from build123d import *

# Parameters (mm, degrees)
CHAMFER1_SIZE    = 0.79375
CHAMFER1_SIZE2   = 3.175
EXTRUSION1_DEPTH = 3.175
ESQUISSE3_R      = 9.165435523
EXTRUSION2_DEPTH = 1.5875
ESQUISSE4_R      = 6.5786
THREAD1_DEPTH    = 4.7625
CHAMFER2_SIZE    = 0.79375
HOLE1_D          = 10.16


with BuildPart() as part:
    # Esquisse1 → Revolution1 (revolve)
    with BuildSketch(Plane.XY, mode=Mode.PRIVATE) as revolution1_sk:
        Polygon((0, 5.08), (19.05, 5.08), (19.05, 6.477), (15.24, 6.477), (15.24, 5.842), (12.7, 6.477), (12.7, 5.842), (10.16, 6.477), (10.16, 5.842), (7.62, 6.477), (7.62, 5.842), (5.08, 6.477), (4.7625, 6.477), (4.7625, 5.842), (0, 5.842), align=None)
    revolve(revolution1_sk.sketch.rotate(Axis((0, 0, 0), (1, 0, 0)), 90), axis=Axis((0, 0, 0), (1, 0, 0)))

    # Chamfer1
    chamfer1_edges = [part.edges().sort_by_distance(p)[0] for p in [
        (19.05, 0, -6.477),
    ]]
    chamfer1_side = [part.faces().sort_by_distance(p)[0] for p in [
        (19.05, 0, -5.263197225),
    ]]
    chamfer(chamfer1_edges, length=CHAMFER1_SIZE, length2=CHAMFER1_SIZE2, reference=chamfer1_side[0])

    # Esquisse2 → Extrusion1 (add)
    with BuildSketch(Plane.ZY):
        Polygon((0.375877143, -9.157724865), (-7.742883803, -4.904381587), (-8.118760946, 4.253343278), (-0.375877143, 9.157724865), (7.742883803, 4.904381587), (8.118760946, -4.253343278), align=None)
    extrude(amount=EXTRUSION1_DEPTH)

    # Esquisse3 → Extrusion2 (add)
    with BuildSketch(Plane.ZY.offset(3.175)):
        with Locations(Location((0, 0, 0), (0, 0, 152.350375514))):
            Circle(ESQUISSE3_R)
    extrude(amount=EXTRUSION2_DEPTH)

    # Esquisse4 → Thread1 (add)
    with BuildSketch(Plane.ZY.offset(4.7625)):
        with Locations(Location((0, 0, 0), (0, 0, 180))):
            Circle(ESQUISSE4_R)
    extrude(amount=THREAD1_DEPTH)

    # Chamfer2
    chamfer2_edges = [part.edges().sort_by_distance(p)[0] for p in [
        (-9.525, 0, 6.5786),
    ]]
    chamfer(chamfer2_edges, length=CHAMFER2_SIZE)

    # Hole1 (through all)
    with Locations(Plane.ZY.offset(9.525)):
        with Locations((0, 0)):
            Hole(HOLE1_D / 2)


solid = part.part
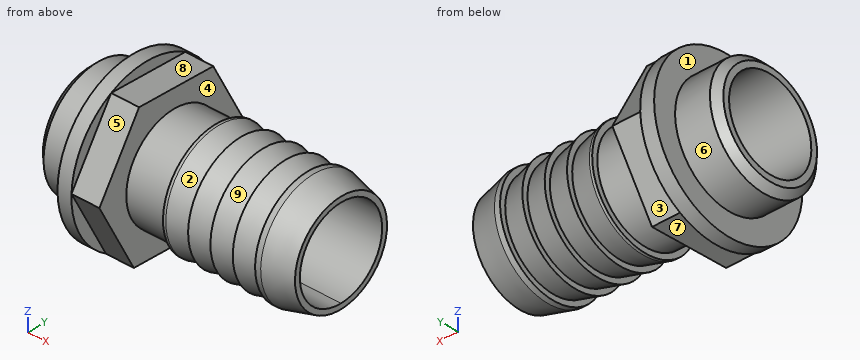
Could you check a few things on this model? Use its own coordinates, in mm. Face numbers are marked on the shaded views. A direction names the side the tool comes from. Round coordinates to 2 decimals unless told otherwise and drop trailing zeros. Loops run counter-clockwise (first coordinate to the right, second up) from the corner with the lowest first, then second, coordinate; pieces in that order, holes last. Notation, with made-up numbers: (39.5, -27.75) - (61.5, -27.75) arc R25 ccw to (61.5, 6.25) - close; hole circle Ø1 at (47, 52). An arc over 180 degrees is marked (long way). Write item = value, one per line.
1) I need wall thicknesses on line 1 along Y through (x, z) = (-5.5, 0); line 2 along X through (y, z) = (0.5, 8) (1 decimal); line 3 along X through (y, z) = (-6.25, -4). Which ranges of each line are inside material? Lowest first, please. Write a range as from..to.
Computed:
line_1 = -6.58..-5.08, 5.08..6.58
line_2 = -4.8..-3.2
line_3 = -4.76..0
2) Imagine slicing it at B-B (y = -8). Please give me the cut outline in (x, z) (1 decimal), and give its area (3 significant figures).
Computed:
outline = (-4.8, -4.5) - (-3.2, -4.5) - (-3.2, -1.8) - (0, -1.8) - (0, 2.2) - (-3.2, 2.2) - (-3.2, 4.5) - (-4.8, 4.5) - close
area = 27.0 mm2
3) I'm going to push flat-ended pins straight in: P1, Ø1, axis at x = 10.5, y = -1.5, coming from the -Z side; P2, Ø4, axis at y = 3, z = -1, coming from the -X side (3 decimals); P3, Ø5, axis at x = 6, z = 4.5, coming from the -Y side; P4, Ø4, axis at x = 15.5, y = 7, coming from the +Z side. Where does each tip first touch, or does it pass through?
Computed:
P1 = -6.38
P2 = -9.525
P3 = -6.1
P4 = 4.12
4) If we mould it in two halves opening along X, with no side actions, what happens to the marked faces 1, 2, 3 and 4? For each: pulls with the +X half, pulls with the -X half, needs draft (parallel to the pull), parting line crosses it, or undercut.
Computed:
face_1 = pulls with the -X half
face_2 = undercut
face_3 = needs draft
face_4 = undercut
5) Imagine slicing it at A-A (z = -7). Please give me the cut outline in (x, y) (1 decimal).
Computed:
outline = (-4.8, -5.9) - (-3.2, -5.9) - (-3.2, -5.3) - (0, -5.3) - (0, 5) - (-3.2, 5) - (-3.2, 5.9) - (-4.8, 5.9) - close
6) On a 3-axis mill with a long thin cutter (end or side, diameter ignored), from which of +Z, -Z, +X, -X, +Y, -Y can I reach the whole of each face in a straight line? I mean the marked faces 5, 6, 7, 8 and 9. Say none if no direction works.
Computed:
face_5 = +Z, +X, -Y
face_6 = -X
face_7 = -Z, +X, -Y
face_8 = +Z, +X, +Y
face_9 = none
